from build123d import *

# Parameters (mm, degrees)
SKETCH1_R             = 4.5640625
BOSS_EXTRUDE1_DEPTH   = 2.9765625
SKETCH2_R             = 4.7625
BOSS_EXTRUDE2_DEPTH   = 12.7
FILLET1_R             = 3.175
FILLET2_R             = 2.976563
SKETCH3_W             = 2.495765829
SKETCH3_H             = 5.953125
CUT_EXTRUDE1_DEPTH    = 25.4
F_6_32_TAPPED_HOLE1_D = 3.5052


with BuildPart() as part:
    # Sketch1 → Boss-Extrude1 (new, symmetric)
    with BuildSketch(Plane.XY):
        with BuildLine():
            Line((34.572359171, 0), (34.572359171, 50.8))
            Line((34.572359171, 50.8), (55.121390829, 50.8))
            Line((55.121390829, 50.8), (55.121390829, 0))
            ThreePointArc((55.121390829, 0), (44.846875, -10.274515829), (34.572359171, 0))
        make_face()
        with Locations((44.846875, 0)):
            Circle(SKETCH1_R, mode=Mode.SUBTRACT)
    extrude(amount=BOSS_EXTRUDE1_DEPTH, both=True)

    # Sketch2 → Boss-Extrude2 (add, symmetric)
    with BuildSketch(Plane.XY):
        with Locations((44.846875, 0)):
            Circle(SKETCH2_R)
    extrude(amount=BOSS_EXTRUDE2_DEPTH, both=True)

    # Fillet1
    fillet1_edges = [part.edges().sort_by_distance(p)[0] for p in [
        (40.084375, 0, -12.7),
        (40.084375, 0, 12.7),
    ]]
    fillet(fillet1_edges, radius=FILLET1_R)

    # Fillet2
    fillet2_edges = [part.edges().sort_by_distance(p)[0] for p in [
        (34.572359171, 25.4, 2.9765625),
        (44.846875, -10.274515829, 2.9765625),
        (34.572359171, 25.4, -2.9765625),
        (55.121390829, 25.4, -2.9765625),
        (55.121390829, 25.4, 2.9765625),
    ]]
    fillet(fillet2_edges, radius=FILLET2_R - 0.0001)  # a hair under: the kernel refuses the full size

    # Sketch3 → Cut-Extrude1 (cut)
    with BuildSketch(Plane(origin=(0, 50.8, 0), x_dir=(1, 0, 0), z_dir=(0, 1, 0))):
        with Locations((35.820242085, 0)):
            Rectangle(SKETCH3_W, SKETCH3_H)
    extrude(amount=-CUT_EXTRUDE1_DEPTH, mode=Mode.SUBTRACT)

    # #6-32 Tapped Hole1 (through all)
    with Locations(Plane(origin=(0, 0, -2.9765625), x_dir=(-1, 0, 0), z_dir=(0, 0, -1))):
        with Locations((-44.846875, 41.021), (-44.846875, 31.242)):
            Hole(F_6_32_TAPPED_HOLE1_D / 2)


solid = part.part
Geometry check sheet. Reference: the model listing, model coordinates, mm. A direction names the side the tool comes from. Give positions to 0.01 mm unless a question says otherwise; leave off trailing zeros. Order: outer loops, then holes, each group sorted by start corner. A loop starts at its lowest first (then second) coordinate and runs counter-clockwise, first axis right, second up. Notation, with made-up numbers: (34, 79) - (71, 79) arc R15 ccw to (71, 87) - close; hole circle Ø4 at (-16.75, 64.5). An arc over 180 degrees is marked (long way). Use one line per item in the form item = value.
1) Sectioned sample at C-C (z = -7.5). Record the boundary of the cut face in (x, y) (1 decimal), and give its area (3 significant figures).
Working result:
outline = circle Ø9.5 at (44.8, 0)
area = 71.3 mm^2
2) Access from +Z, -Z, +X, -X, +Y, -Y to the whole of each face (thin tool, end or side, straight path). Record for faces 1 (the face through (37.068, 38, 0)), 2 (the face through (54.226, 25.044, -2.128)), 3 (the face through (49.4, 1.4, -6.2)).
Working result:
face_1 = +Z, -Z, -X, +Y
face_2 = -Z, +X, +Y, -Y
face_3 = -Z
3) Depth check by flat-ended pin: pin 1 Ø12 at (x, y) = (39, 25) entering from +Z; pin 2 Ø6.5 at (y, z) = (36.5, -0.5) entering from -X; pin 3 Ø1.5 at (x, z) = (49, -6.5) entering from -Y. Enter the tip coordinate at first touch or a pass-through.
Working result:
pin_1 = 2.98
pin_2 = 37.07
pin_3 = -3.33
4) Material ranges on probe 1 along Y at (x, z) = (44.75, 1.5); probe 2 along Z at (x, y) = (41.5, 41); probe 3 along X at (y, z) = (41.5, 0.5), recorded low to high. Write a range as from..to.
Working result:
probe_1 = -9.87..29.49, 32.99..39.27, 42.77..50.8
probe_2 = -2.98..2.98
probe_3 = 37.07..43.16, 46.53..55.08
5) Draft check along Y on faces 4 (the face through (46, 50.8, 0)), 5 (the face through (45.66, 39.47, 0.04)), 6 (the face through (49.4, 1.4, 6.3)), 7 (the face through (46.466, 30.571, 0.042)). Enter one of: released by +Y, released by -Y, zero draft, split by the parting line, or undercut.
Working result:
face_4 = released by +Y
face_5 = undercut
face_6 = split by the parting line
face_7 = undercut
